Print and shaded views of the part. All mm, measured from the part's lowest x, y and z. Coordinates: 2 decimals unless noted, no trailing zeros. Loops run counter-clockwise (first coordinate to the right, second up) from the corner with the lowest first, then second, coordinate; pieces in that order, holes last. Notation, with made-up numbers: M -12.5,0 L 1.5,0 A4 cw 1.5,6 Z; hole C 17,89 d11. An arc over 180 degrees is marked long. Answer as a JSON object with one key per item and string values. Group by question number.
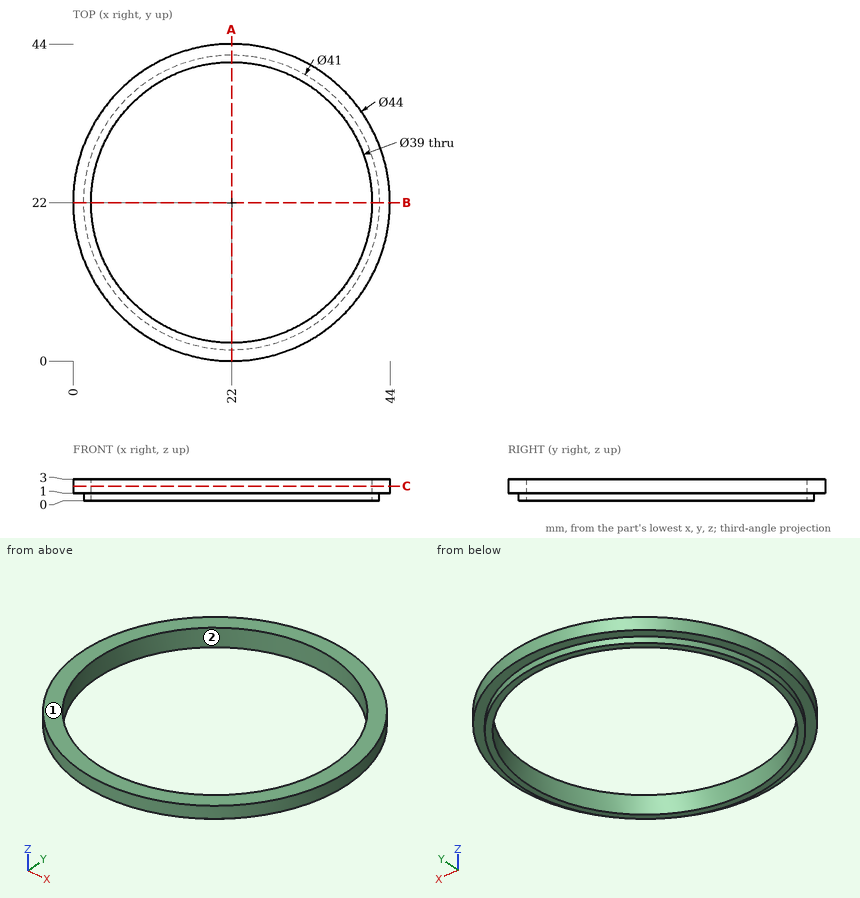
Item 1: Slice it at A-A, the plane x = 22. Write the cut outline in (y, z), then the cut area to 3 significant figures.
Item 2: Slice it at C-C, the plane z = 2. Write the cut outline in (x, y).
Item 3: Pin check, flat tips, straight feed: pin 1 (1.5 mm diameter, centred on y = 28.5, z = 2, fed in from +X); pin 2 (1 mm diameter, centred on y = 5, z = 2, fed in from -X). Stop position of each tip, or through.
Item 4: Pull direction X, two halves, no side cores. Call the marked faces 1 and 2: released by +X, released by -X, zero draft, split by the parting line, or undercut.
Item 5: Drill centre lines: L1, parallel to Y at x = 22, z = 2; L2, parallel to Y at x = 22, z = 0.75; L3, parallel to X at y = 6, z = 0.65. Where is each one in solid material? Low to high. Write a range as from..to.
Computed:
{
 "1": {"outline": "M 0,1 L 1.5,1 L 1.5,0 L 2.5,0 L 2.5,3 L 0,3 Z; M 41.5,0 L 42.5,0 L 42.5,1 L 44,1 L 44,3 L 41.5,3 Z", "area": "12.0 mm2"},
 "2": {"outline": "C 22,22 d44; hole C 22,22 d39"},
 "3": {"pin 1": "x = 43.24", "pin 2": "x = 7.45"},
 "4": {"face 1": "zero draft", "face 2": "undercut"},
 "5": {"L1": "0..2.5, 41.5..44", "L2": "1.5..2.5, 41.5..42.5", "L3": "9.18..10.85, 33.15..34.82"}
}
